```python
from build123d import *

# Parameters (mm, degrees)
F0_W     = 5
F0_H     = 44
F2_SIZE  = 1
F3_DEPTH = 32.5
F4_DEPTH = 31.5


with BuildPart() as f1:
    # F0 (on Front) → F1 (revolve)
    with BuildSketch(Plane.XZ):
        with Locations((-2.5, 36.5)):
            Rectangle(F0_W, F0_H)
        with BuildLine():
            Line((-5, 58.5), (0, 58.5))
            Line((0, 58.5), (0, 92.7705098312))
            ThreePointArc((0, 92.7705098312), (-17.3166671454, 77.7969775189), (-5, 58.5))
        make_face()
    revolve(axis=Axis((0, 0, 75.6352549156), (0, 0, -1)))

    # F0 (on Front) → F3 (join, symmetric)
    with BuildSketch(Plane.XZ):
        Polygon((-31.5, 12.5), (31.5, 12.5), (48.5, 12.5), (48.5, 14.5), (0, 14.5), (-5, 14.5), (-48.5, 14.5), (-48.5, 12.5), align=None)
    extrude(amount=F3_DEPTH, both=True)



with BuildPart() as f1b:
    # F0 (on Front) → F1, piece 2 (revolve)
    with BuildSketch(Plane.XZ):
        Polygon((0, -26.5), (0, -12.5), (-6, -12.5), (-6, -24.5), (-5, -24.5), (-5, -26.5), align=None)
    revolve(axis=Axis((0, 0, 75.6352549156), (0, 0, -1)))

    # F2
    f2_edges = [f1b.edges().sort_by_distance(p)[0] for p in [
        (5, 0, -26.5),
    ]]
    chamfer(f2_edges, length=F2_SIZE)


with BuildPart() as f1_1:
    add(f1.part)

    add(f1b.part)  # F4 merges F1b
    # F0 (on Front) → F4 (join, symmetric)
    with BuildSketch(Plane.XZ):
        Polygon((0, -12.5), (31.5, -12.5), (31.5, 12.5), (-31.5, 12.5), (-31.5, -12.5), (-6, -12.5), align=None)
    extrude(amount=F4_DEPTH, both=True)


solid = f1_1.part
```
Source: CAD feature listing. Evaluate the final solid. Frame: model axes, mm. A direction names the side the tool comes from. Give positions to 0.01 mm unless a question says otherwise; leave off trailing zeros. Order: outer loops, then holes, each group sorted by start corner. A loop starts at its lowest first (then second) coordinate and runs counter-clockwise, first axis right, second up.
(1) Material intervals for line 1 along Z through (x, y) = (33, -20.5); line 2 along Y through (x, z) = (-27.5, -4); line 3 along Z through (x, y) = (25, 0.5), sorted ascending.
(2) Pull-direction query (Z, two-part tool) for faces 1 (the face through (0, 0, -26.5)), 2 (the face through (1.08, -4.88, 36.81)), 3 (the face through (1.08, -4.88, -25.01)); classes: +Z half, -Z half, draft (parallel to the pull), parting line (faces both ways), or undercut.
(3) Section query B-B (x = -12). Return the cut outline in (y, z).
(4) Section query A-A (y = -14). Return the cut outline in (x, z).
(5) Section query D-D (z = 31.5). Return the cut outline in (x, y).
(6) Access query for faces 4 (the face through (0, -31.5, 0)), 5 (the face through (0, 31.5, 0)), 6 (the face through (6, 0, -19)), 7 (the face through (-31.5, 0, 0)). Directions: +Z, -Z, +X, -X, +Y, -Y. A direction counts if a zero-diameter tool reaches every point of the face in a straight line with its end or side. Return the directions, or none.
(7) Contact query for flat-ended pins moving along their axis: P1, Ø19, axis at x = -7, y = -3, coming from the -Z side; P2, Ø20, axis at y = -12.5, z = -5, coming from the -X side; P3, Ø12, axis at x = 7.5, y = 9.5, coming from the +Z side; P4, Ø12, axis at x = -23.5, z = -4, coming from the +Y side. Output: stop coordinate, or through.
(8) Section query C-C (x = 29.5). Return the cut outline in (y, z).
Outcome:
1. line 1: z = 12.5 to 14.5
1. line 2: y = -31.5 to 31.5
1. line 3: z = -12.5 to 14.5
2. face 1: -Z half
2. face 2: undercut
2. face 3: draft
3. outline: (-32.5, 12.5) - (-31.5, 12.5) - (-31.5, -12.5) - (31.5, -12.5) - (31.5, 12.5) - (32.5, 12.5) - (32.5, 14.5) - (-32.5, 14.5) - close; circle Ø25.48 at (0, 75.27)
4. outline: (-48.5, 12.5) - (-31.5, 12.5) - (-31.5, -12.5) - (31.5, -12.5) - (31.5, 12.5) - (48.5, 12.5) - (48.5, 14.5) - (-48.5, 14.5) - close; circle Ø21 at (0, 75.27)
5. outline: circle Ø10 at (0, 0)
6. face 4: -Z, +X, -X, -Y
6. face 5: -Z, +X, -X, +Y
6. face 6: -Z
6. face 7: -Z, -X, +Y, -Y
7. P1: stops at z = -26.5
7. P2: stops at x = -31.5
7. P3: stops at z = 91.67
7. P4: stops at y = 31.5
8. outline: (-32.5, 12.5) - (-31.5, 12.5) - (-31.5, -12.5) - (31.5, -12.5) - (31.5, 12.5) - (32.5, 12.5) - (32.5, 14.5) - (-32.5, 14.5) - close
